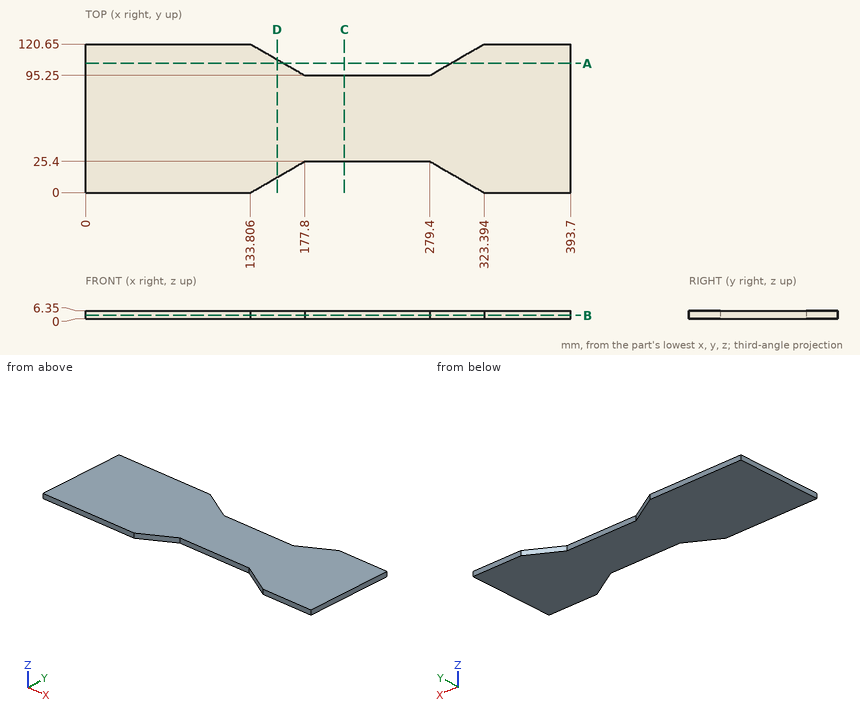
The figure shows three views and two pictorial views of one solid part (mm, origin at its lowest corner). Answer the questions. Round coordinates to 2 decimals unless told otherwise and drop trailing zeros. Write each loop counter-clockwise with the first axis right and the second up, starting at its lowest first coordinate (ties: lowest second). Pieces come first, ordered by that corner, then holes. Notation, with made-up numbers: (38, 18.25) -> (89, 18.25) arc R21 cw to (89, 27.25) -> close; hole circle Ø9 at (-20, 30.25). An arc over 180 degrees is marked (long way). Write each question's results on one line, items separated by ' | '.
Q1. Straight lines are drawn through the part: line 1 along Y through (x, z) = (190, 2.5); line 2 along X through (y, z) = (99, 5.25) (1 decimal); line 3 along X through (y, z) = (25, 2.25). For each, find the intervals that lie inside material, in ascending order. Write a range as [from, to].
Data:
line 1: [25.4, 95.25] | line 2: [0, 171.3], [285.9, 393.7] | line 3: [0, 177.11], [280.09, 393.7]
Q2. Section A-A, the plane y = 105 is taken. Write down the section's boundary in (x, z), then the cut area to 3 significant figures.
Data:
outline: (0, 0) -> (160.91, 0) -> (160.91, 6.35) -> (0, 6.35) -> close; (296.29, 0) -> (393.7, 0) -> (393.7, 6.35) -> (296.29, 6.35) -> close | area: 1,640 mm^2
Q3. Flat-ended cylindrical pins translate along their axes: P1, Ø3, axis at x = 250, z = 2.5, coming from the +Y side; P2, Ø1.5, axis at x = 202.5, z = 5.5, coming from the -Y side. Find the tip coordinate at first contact, or state that the pin passes through.
Data:
P1: y = 95.25 | P2: y = 25.4
Q4. Section D-D, the plane x = 155.5 is taken. Write down the section's boundary in (y, z) (3 decimals), then the cut area to 3 significant figures.
Data:
outline: (12.525, 0) -> (108.125, 0) -> (108.125, 6.35) -> (12.525, 6.35) -> close | area: 607 mm^2
Q5. Section C-C, the plane x = 210 is taken. Write down the section's boundary in (y, z), then the cut area to 3 significant figures.
Data:
outline: (25.4, 0) -> (95.25, 0) -> (95.25, 6.35) -> (25.4, 6.35) -> close | area: 444 mm^2
Q6. Section B-B, the plane z = 2.5 is taken. Write down the section's boundary in (x, y), then the cut area to 3 significant figures.
Data:
outline: (0, 0) -> (133.81, 0) -> (177.8, 25.4) -> (279.4, 25.4) -> (323.39, 0) -> (393.7, 0) -> (393.7, 120.65) -> (323.39, 120.65) -> (279.4, 95.25) -> (177.8, 95.25) -> (133.81, 120.65) -> (0, 120.65) -> close | area: 40,100 mm^2
